Input: part model. Units: mm. Frame: model coordinates. Give positions to 0.01 mm unless a question says otherwise; leave off trailing zeros. Write each loop counter-clockwise with the first axis right and the second up, starting at its lowest first coordinate (ties: lowest second). Pieces come first, ordered by that corner, then holes. Notation, with made-up numbers: (44, -20) - (48, -20) arc R14 ccw to (48, -6) - close; hole circle Ø9 at (34, 44). An arc over 180 degrees is marked (long way). Answer as CSV lines item,"result".
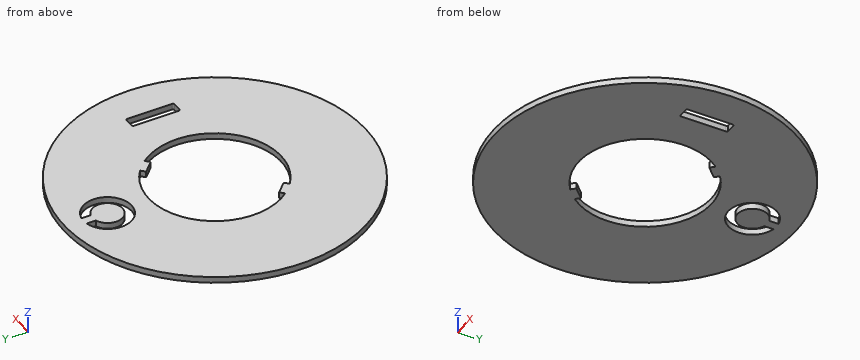
```python
from build123d import *

# Parameters (mm, degrees)
SKETCH1_R           = 25
BOSS_EXTRUDE1_DEPTH = 1.016
CUT_EXTRUDE1_DEPTH  = 158.985038077


with BuildPart() as part:
    # Sketch1 → Boss-Extrude1 (new body)
    with BuildSketch(Plane.XY):
        with Locations((107.000000001, 61.8)):
            Circle(SKETCH1_R)
        with BuildLine():
            Line((113.843907282, 70.411674235), (113.187184336, 69.754951288))
            Line((113.187184336, 69.754951288), (114.954951289, 67.987184335))
            Line((114.954951289, 67.987184335), (115.611674235, 68.643907282))
            ThreePointArc((115.611674235, 68.643907282), (114.778174594, 54.021825407), (100.156092719, 53.188325765))
            Line((100.156092719, 53.188325765), (100.812815665, 53.845048712))
            Line((100.812815665, 53.845048712), (99.045048712, 55.612815665))
            Line((99.045048712, 55.612815665), (98.388325766, 54.956092718))
            ThreePointArc((98.388325766, 54.956092718), (99.221825408, 69.578174593), (113.843907282, 70.411674235))
        make_face(mode=Mode.SUBTRACT)
    extrude(amount=BOSS_EXTRUDE1_DEPTH)

    # Sketch2 → Cut-Extrude1 (cut, through all)
    with BuildSketch(Plane.XY):
        with BuildLine():
            ThreePointArc((106.250000001, 82.184848004), (107.000000001, 77.3), (107.750000001, 82.184848004))
            Line((107.750000001, 82.184848004), (107.750000001, 83.729058411))
            ThreePointArc((107.750000001, 83.729058411), (107.000000001, 75.8), (106.250000001, 83.729058411))
            Line((106.250000001, 83.729058411), (106.250000001, 82.184848004))
        make_face()
        with BuildLine():
            ThreePointArc((124.000000001, 65.55), (124.073223305, 65.726776695), (124.250000001, 65.8))
            Line((124.250000001, 65.8), (125.750000001, 65.8))
            ThreePointArc((125.750000001, 65.8), (125.926776696, 65.726776695), (126.000000001, 65.55))
            Line((126.000000001, 65.55), (126.000000001, 58.05))
            ThreePointArc((126.000000001, 58.05), (125.926776696, 57.873223305), (125.750000001, 57.8))
            Line((125.750000001, 57.8), (124.250000001, 57.8))
            ThreePointArc((124.250000001, 57.8), (124.073223305, 57.873223305), (124.000000001, 58.05))
            Line((124.000000001, 58.05), (124.000000001, 65.55))
        make_face()
    extrude(amount=CUT_EXTRUDE1_DEPTH, mode=Mode.SUBTRACT)


solid = part.part
```
Item 1: Cut plane D-D on x = 117. Return the cut outline in (y, z), plus the area to 3 significant figures.
The answers:
outline,"(38.89, 0) - (57.22, 0) - (57.22, 1.02) - (38.89, 1.02) - close; (66.38, 0) - (84.71, 0) - (84.71, 1.02) - (66.38, 1.02) - close"
area,"37.2 mm²"
Item 2: Cut plane A-A on x = 107. Return the cut outline in (y, z).
The answers:
outline,"(36.8, 0) - (50.8, 0) - (50.8, 1.02) - (36.8, 1.02) - close; (72.8, 0) - (75.8, 0) - (75.8, 1.02) - (72.8, 1.02) - close; (77.3, 0) - (86.8, 0) - (86.8, 1.02) - (77.3, 1.02) - close"
Item 3: Cut plane B-B on y = 61.8. Return the cut outline in (x, z), plus the area to 3 significant figures.
The answers:
outline,"(82, 0) - (96, 0) - (96, 1.02) - (82, 1.02) - close; (118, 0) - (124, 0) - (124, 1.02) - (118, 1.02) - close; (126, 0) - (132, 0) - (132, 1.02) - (126, 1.02) - close"
area,"26.4 mm²"
Item 4: Ray query, line 1 (X direction, y = 59, z = 0.65); line 2 (X direction, y = 63, z = 0.9); line 3 (Y direction, x = 110, z = 0.9). Return the intervals inside material, ascending. Write a range as from..to.
The answers:
line 1,"82.16..96.36, 117.64..124, 126..131.84"
line 2,"82.03..96.07, 117.93..124, 126..131.97"
line 3,"36.98..51.22, 72.38..77.15, 82.45..86.62"
Item 5: Cut plane C-C on z = 0.25. Return the cut outline in (x, y).
The answers:
outline,"circle Ø50 at (107, 61.8); hole (98.39, 54.96) - (99.05, 55.61) - (100.81, 53.85) - (100.16, 53.19) arc R11 ccw to (115.61, 68.64) - (114.95, 67.99) - (113.19, 69.75) - (113.84, 70.41) arc R11 ccw to start; hole (106.25, 82.18) - (106.25, 83.73) arc R4 ccw (long way) to (107.75, 83.73) - (107.75, 82.18) arc R2.5 cw (long way) to start; hole (124, 58.05) arc R0.25 ccw to (124.25, 57.8) - (125.75, 57.8) arc R0.25 ccw to (126, 58.05) - (126, 65.55) arc R0.25 ccw to (125.75, 65.8) - (124.25, 65.8) arc R0.25 ccw to (124, 65.55) - close"
Item 6: Contact query for flat-ended pins moving along their axis: pin 1 (0.5 mm diameter, centred on x = 125, z = 0.5, fed in from -Y); pin 2 (0.5 mm diameter, centred on y = 63, z = 0.5, fed in from -X); pin 3 (3 mm diameter, centred on x = 110.5, y = 53.5, fed in from +Z). Output: stop coordinate, or through.
The answers:
pin 1,"y = 44.19"
pin 2,"x = 82.02"
pin 3,"through"
